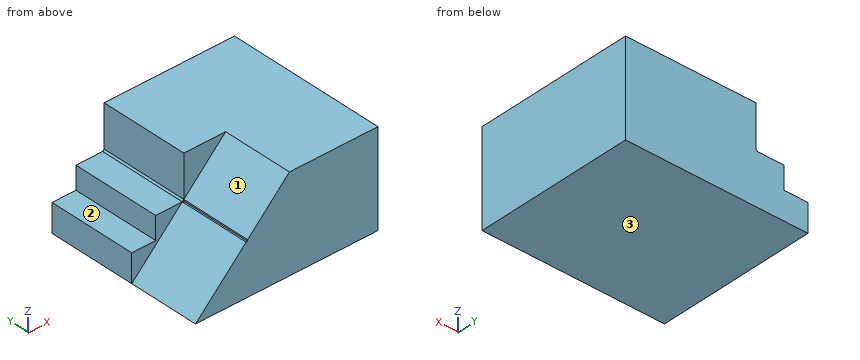
```python
from build123d import *

# Parameters (mm, degrees)
F1_DEPTH = 20.32
F2_DEPTH = 25.4
F3_DEPTH = 25.4


with BuildPart() as f1:
    # F0 (on Front) → F1 (new body)
    with BuildSketch(Plane.XZ):
        Polygon((14.508714, 14.508714), (0, 0), (26.940768, 0), (26.940768, 26.940768), (14.94181, 14.94181), (14.94181, 14.508714), align=None)
    extrude(amount=F1_DEPTH)

    # F0 (on Front) → F2 (join)
    with BuildSketch(Plane.XZ):
        Polygon((14.508714, 14.508714), (0, 0), (26.940768, 0), (26.940768, 26.940768), (14.94181, 14.94181), (14.94181, 14.508714), align=None)
        Polygon((0, 8.012275), (0, 0), (14.508714, 14.508714), (6.857352, 14.508714), (6.857352, 8.012275), align=None)
        Polygon((14.94181, 14.94181), (14.508714, 14.508714), (14.94181, 14.508714), align=None)
        Polygon((14.94181, 14.94181), (26.940768, 26.940768), (14.94181, 26.940768), align=None)
    extrude(amount=-F2_DEPTH)

    # F2_face (on face) → F3 (join)
    with BuildSketch(Plane(origin=(26.940768, 2.54, 13.470384), x_dir=(0, 1, 0), z_dir=(1, 0, 0))):
        Polygon((-22.86, -13.470384), (22.86, -13.470384), (22.86, 13.470384), (-2.54, 13.470384), (-22.86, 13.470384), align=None)
    extrude(amount=F3_DEPTH)


solid = f1.part
```
The listing builds one solid part. Answer for the finished solid, in the listing's coordinates (mm). Face numbers are marked on the shaded views. A direction names the side the tool comes from. Give positions to 0.01 mm unless a question says otherwise; leave off trailing zeros. Order: outer loops, then holes, each group sorted by start corner. A loop starts at its lowest first (then second) coordinate and runs counter-clockwise, first axis right, second up. Notation, with made-up numbers: (84, 78) - (102, 78) arc R30 cw to (102, 108) - close; hole circle Ø5 at (-28.75, 57). An arc over 180 degrees is marked (long way). Answer in a Markdown table with one row per item. Add a question column.
Q1. Find the intervals of material crossed by line 1 along X through (y, z) = (11.5, 8.5); line 2 along Y through (x, z) = (12, 13.75); line 3 along X through (y, z) = (-17.5, 25.75), in increasing order. Write a range as [from, to].
Q2. Given P1, Ø0.5, axis at y = -7, z = 14.5, coming from the -X side; P2, Ø8, axis at x = 40, y = 2.5, coming from the -Z side; P3, Ø3.5, axis at y = 14.5, z = 19.5, coming from the -X side; P4, Ø8.5, axis at x = 10.5, y = 16.5, coming from the +Z side, each flat-ended and moving along its own axis, determine where each tip first touches the part or whether it passes through.
Q3. The part is cut by section D-D (y = -8). Determine the outline of the cut face in (x, z), then the cut area to 3 significant figures.
Q4. The part is cut by section B-B (z = 9.25). Determine the outline of the cut face in (x, y), then the cut area to 3 significant figures.
Q5. The part is cut by section A-A (y = 1). Determine the outline of the cut face in (x, z).
Q6. The part is cut by section C-C (x = 8). Determine the outline of the cut face in (y, z), then the cut area to 3 significant figures.
Q7. Which of the six approach directions +Z, -Z, +X, -X, +Y, -Y give full straight-line access (tool end or side, diameter ignored) to the marked faces 1, 2 and 3?
Determined:
| question | item | result |
|---|---|---|
| 1 | line 1 | x = [6.86, 52.34] |
| 1 | line 2 | y = [0, 25.4] |
| 1 | line 3 | x = [25.75, 52.34] |
| 2 | P1 | stops at x = 14.25 |
| 2 | P2 | stops at z = 0 |
| 2 | P3 | stops at x = 14.94 |
| 2 | P4 | stops at z = 14.75 |
| 3 | outline | (0, 0) - (52.34, 0) - (52.34, 26.94) - (26.94, 26.94) - (14.94, 14.94) - (14.94, 14.51) - (14.51, 14.51) - close |
| 3 | area | 1,050 mm² |
| 4 | outline | (6.86, 0) - (9.25, 0) - (9.25, -20.32) - (52.34, -20.32) - (52.34, 25.4) - (6.86, 25.4) - close |
| 4 | area | 2,030 mm² |
| 5 | outline | (0, 0) - (52.34, 0) - (52.34, 26.94) - (14.94, 26.94) - (14.94, 14.94) - (14.51, 14.51) - (6.86, 14.51) - (6.86, 8.01) - (0, 8.01) - close |
| 6 | outline | (-20.32, 0) - (25.4, 0) - (25.4, 14.51) - (0, 14.51) - (0, 8) - (-20.32, 8) - close |
| 6 | area | 531 mm² |
| 7 | face 1 | +Z, -X, -Y |
| 7 | face 2 | +Z, -X, +Y, -Y |
| 7 | face 3 | -Z, +X, -X, +Y, -Y |
